```python
from build123d import *

# Parameters (mm, degrees)
SKETCH_1_W      = 2
SKETCH_1_H      = 1
SKETCH_1_W_2    = 3
SKETCH_1_W_3    = 1
EXTRUDE_1_DEPTH = 1
SKETCH_1_3_W    = 3
SKETCH_1_3_H    = 1
EXTRUDE_2_DEPTH = 2
SKETCH_1_4_W    = 2
SKETCH_1_4_H    = 1
EXTRUDE_3_DEPTH = 3
SKETCH_1_5_W    = 1
SKETCH_1_5_H    = 1
EXTRUDE_4_DEPTH = 5
FILLET_1_R      = 1
EXTRUDE_5_DEPTH = 1


with BuildPart() as part:
    # 草圖1 → 填料-伸長1 (new body)
    with BuildSketch(Plane(origin=(0, 0, 0), x_dir=(1, 0, 0), z_dir=(0, 1, 0))):
        with Locations((1, 4.5)):
            Rectangle(SKETCH_1_W, SKETCH_1_H)
        with BuildLine():
            Line((0, 4), (0, 0))
            Line((0, 0), (2, 0))
            ThreePointArc((2, 0), (2.707106781, 0.292893219), (3, 1))
            Line((3, 1), (3, 3))
            Line((3, 3), (5, 3))
            ThreePointArc((5, 3), (5.707106781, 3.292893219), (6, 4))
            Line((6, 4), (5, 4))
            Line((5, 4), (2, 4))
            Line((2, 4), (0, 4))
        make_face()
        with Locations((3.5, 4.5)):
            Rectangle(SKETCH_1_W_2, SKETCH_1_H)
        with Locations((5.5, 4.5)):
            Rectangle(SKETCH_1_W_3, SKETCH_1_H)
    extrude(amount=EXTRUDE_1_DEPTH)

    # 草圖1<3> → 填料-伸長2 (add)
    with BuildSketch(Plane(origin=(0, 0, 0), x_dir=(1, 0, 0), z_dir=(0, 1, 0))):
        with Locations((3.5, 4.5)):
            Rectangle(SKETCH_1_3_W, SKETCH_1_3_H)
    extrude(amount=EXTRUDE_2_DEPTH)

    # 草圖1<4> → 填料-伸長3 (add)
    with BuildSketch(Plane(origin=(0, 0, 0), x_dir=(1, 0, 0), z_dir=(0, 1, 0))):
        with Locations((1, 4.5)):
            Rectangle(SKETCH_1_4_W, SKETCH_1_4_H)
    extrude(amount=EXTRUDE_3_DEPTH)

    # 草圖1<5> → 填料-伸長4 (add)
    with BuildSketch(Plane(origin=(0, 0, 0), x_dir=(1, 0, 0), z_dir=(0, 1, 0))):
        with Locations((5.5, 4.5)):
            Rectangle(SKETCH_1_5_W, SKETCH_1_5_H)
    extrude(amount=EXTRUDE_4_DEPTH)

    # 圓角1
    fillet_1_edges = [part.edges().sort_by_distance(p)[0] for p in [
        (6, 5, -4.5),
    ]]
    fillet(fillet_1_edges, radius=FILLET_1_R - 0.0001)  # a hair under: the kernel refuses the full size

    # 草圖2 → 填料-伸長5 (add)
    with BuildSketch(Plane(origin=(0, 0, 0), x_dir=(0, 0, -1), z_dir=(1, 0, 0))):
        Polygon((0, 1), (4, 3), (4, 1), align=None)
    extrude(amount=EXTRUDE_5_DEPTH)


solid = part.part
```
Design review of the part built by this model. Coordinates are the model's own, in mm. A direction names the side the tool comes from. Give positions to 0.01 mm unless a question says otherwise; leave off trailing zeros. Loops run counter-clockwise (first coordinate to the right, second up) from the corner with the lowest first, then second, coordinate; pieces in that order, holes last. Notation, with made-up numbers: M -11.5,63 L 47.5,63 A18 ccw 47.5,96 Z; hole C 50.25,-19.5 d6. An arc over 180 degrees is marked long. Return JSON: item names as keys, results as strings. Group by question number.
Item 1: Tool access review of faces 4 (the flat face through (3.5, 2, -4.5)), 5 (the flat face through (4, 0.5, -3)), 6 (the flat face through (1, 2, -3)), 7 (the flat face through (1, 3, -4.5)), 8 (the flat face through (6, 2, -4.5)): name each direction out of +Z, -Z, +X, -X, +Y, -Y from which nothing blocks a thin tool from reaching the whole face with its end or side.
Item 2: Mouldability with a two-part tool opening along X and no side actions: class faces 1 (the flat face through (0, 1, -3)), 2 (the cylindrical face through (5.699, 4.715, -4.507)), 3 (the flat face through (5, 3.5, -4.5)) as released by +X, released by -X, zero draft, split by the parting line, or undercut.
Item 3: We need section A-A (y = 2.1). Give the boundary of the cut face in (x, z).
Item 4: Insertion check: pin 1 Ø0.5 at (x, z) = (1.5, -4.5) entering from +Y; pin 2 Ø0.8 at (x, y) = (3.5, 0.5) entering from +Z; pin 3 Ø0.8 at (x, z) = (3, -4.5) entering from +Y. Each pin has a flat end and moves straight along its axis. Give the tip position at first contact, or say it passes through.
Item 5: For probe 1 along X at (y, z) = (2.85, -4.8); probe 2 along Z at (x, y) = (5.65, 3.7); probe 3 along X at (y, z) = (1.35, -1), list the stretches that pass through material, from the lowest coordinate up.
Item 6: We need section D-D (y = 2.9). Give the boundary of the cut face in (x, z), and give its area (3 significant figures).
Item 7: We need section B-B (x = 4.4). Give the boundary of the cut face in (y, z), and give its area (3 significant figures).
Item 8: We need section C-C (z = -1.5). Give the boundary of the cut face in (x, y).
Output:
{
 "1": {"face 4": "+Z, -Z, +Y", "face 5": "+Z, +X, +Y, -Y", "face 6": "+Z, +X, +Y", "face 7": "+Z, -Z, -X, +Y", "face 8": "+Z, -Z, +X, +Y, -Y"},
 "2": {"face 1": "released by -X", "face 2": "released by +X", "face 3": "undercut"},
 "3": {"outline": "M 0,-5 L 2,-5 L 2,-4 L 1,-4 L 1,-2.2 L 0,-2.2 Z; M 5,-5 L 6,-5 L 6,-4 L 5,-4 Z"},
 "4": {"pin 1": "stops at y = 3", "pin 2": "stops at z = -3", "pin 3": "stops at y = 2"},
 "5": {"probe 1": "x = 0 to 2, 5 to 6", "probe 2": "z = -5 to -4", "probe 3": "x = 0 to 1"},
 "6": {"outline": "M 0,-5 L 2,-5 L 2,-4 L 1,-4 L 1,-3.8 L 0,-3.8 Z; M 5,-5 L 6,-5 L 6,-4 L 5,-4 Z", "area": "3.20 mm^2"},
 "7": {"outline": "M 0,-5 L 2,-5 L 2,-4 L 1,-4 L 1,-3 L 0,-3 Z", "area": "3.00 mm^2"},
 "8": {"outline": "M 0,0 L 3,0 L 3,1 L 1,1 L 1,1.75 L 0,1.75 Z"}
}
